For this review, take the finished solid that the model builds, in its own axes (mm). Give positions to 0.01 mm unless a question says otherwise; leave off trailing zeros. One line per item, written item: value. Start each with the question number.
Item 1: Mouldability with a two-part tool opening along X and no side actions: class faces 1 (the face through (4, -20, 4)), 2 (the face through (-95.39, 144.48, 1.97)), 3 (the face through (-150.994, 155.07, 1.972)) as released by +X, released by -X, zero draft, split by the parting line, or undercut.
Item 2: Clearance check with a flat-ended pin moving along its axis: pin 1 Ø6 at (x, y) = (6, 126.92) entering from +Z. State where the tip first meets the part, or that it passes through.
Item 3: To check wall thickness, follow probe 1 along Y at (x, z) = (96.5, 0.4); probe 2 along Y at (x, z) = (-90, 0.7). State the ranges of each line that lie inside material, in increasing order.
```python
from build123d import *

# Parameters (mm, degrees)
F0_R     = 2.1
F0_R_2   = 10.65
F0_R_3   = 1.6
F0_R_4   = 5
F1_DEPTH = 4


with BuildPart() as f1:
    # F0 (on Top) → F1 (new body)
    with BuildSketch(Plane.XY):
        with BuildLine():
            Line((155.998865, 157.921114), (-144.001135, 157.921114))
            ThreePointArc((-144.001135, 157.921114), (-151.072203, 154.992182), (-154.001135, 147.921114))
            Line((-154.001135, 147.921114), (-154.001135, -192.078886))
            ThreePointArc((-154.001135, -192.078886), (-151.072203, -199.149954), (-144.001135, -202.078886))
            Line((-144.001135, -202.078886), (155.998865, -202.078886))
            ThreePointArc((155.998865, -202.078886), (163.069933, -199.149954), (165.998865, -192.078886))
            Line((165.998865, -192.078886), (165.998865, 147.921114))
            ThreePointArc((165.998865, 147.921114), (163.069933, 154.992182), (155.998865, 157.921114))
        make_face()
        with Locations((-105.314844, 122.607405)):
            Circle(F0_R, mode=Mode.SUBTRACT)
        with Locations((-94.001135, 133.921114)):
            Circle(F0_R_2, mode=Mode.SUBTRACT)
        with Locations((-82.687427, 122.607405)):
            Circle(F0_R, mode=Mode.SUBTRACT)
        with Locations((-105.314844, 145.234822)):
            Circle(F0_R, mode=Mode.SUBTRACT)
        with Locations((-82.687427, 145.234822)):
            Circle(F0_R, mode=Mode.SUBTRACT)
        with Locations((-2.001135, 126.921114)):
            Circle(F0_R_3, mode=Mode.SUBTRACT)
        with Locations((5.998865, 126.921114)):
            Circle(F0_R_4, mode=Mode.SUBTRACT)
        with Locations((13.998865, 126.921114)):
            Circle(F0_R_3, mode=Mode.SUBTRACT)
        with Locations((94.685156, 122.607405)):
            Circle(F0_R, mode=Mode.SUBTRACT)
        with Locations((117.312573, 122.607405)):
            Circle(F0_R, mode=Mode.SUBTRACT)
        with Locations((105.998865, 133.921114)):
            Circle(F0_R_2, mode=Mode.SUBTRACT)
        with Locations((94.685156, 145.234822)):
            Circle(F0_R, mode=Mode.SUBTRACT)
        with Locations((117.312573, 145.234822)):
            Circle(F0_R, mode=Mode.SUBTRACT)
    extrude(amount=F1_DEPTH)


solid = f1.part
```
Model answer:
1. face 1: zero draft
1. face 2: undercut
1. face 3: released by -X
2. pin 1: passes through
3. probe 1: y = -202.08 to 121.55, 123.66 to 129.11, 138.74 to 144.18, 146.29 to 157.92
3. probe 2: y = -202.08 to 124.05, 143.79 to 157.92
